Answer from the drawing. Dimensions are ordinates in mm from the lowest x, y and z of the part. A direction names the side the tool comes from. Round coordinates to 2 decimals unless told otherwise and drop trailing zeros. Loops run counter-clockwise (first coordinate to the right, second up) from the corner with the lowest first, then second, coordinate; pieces in that order, holes last.
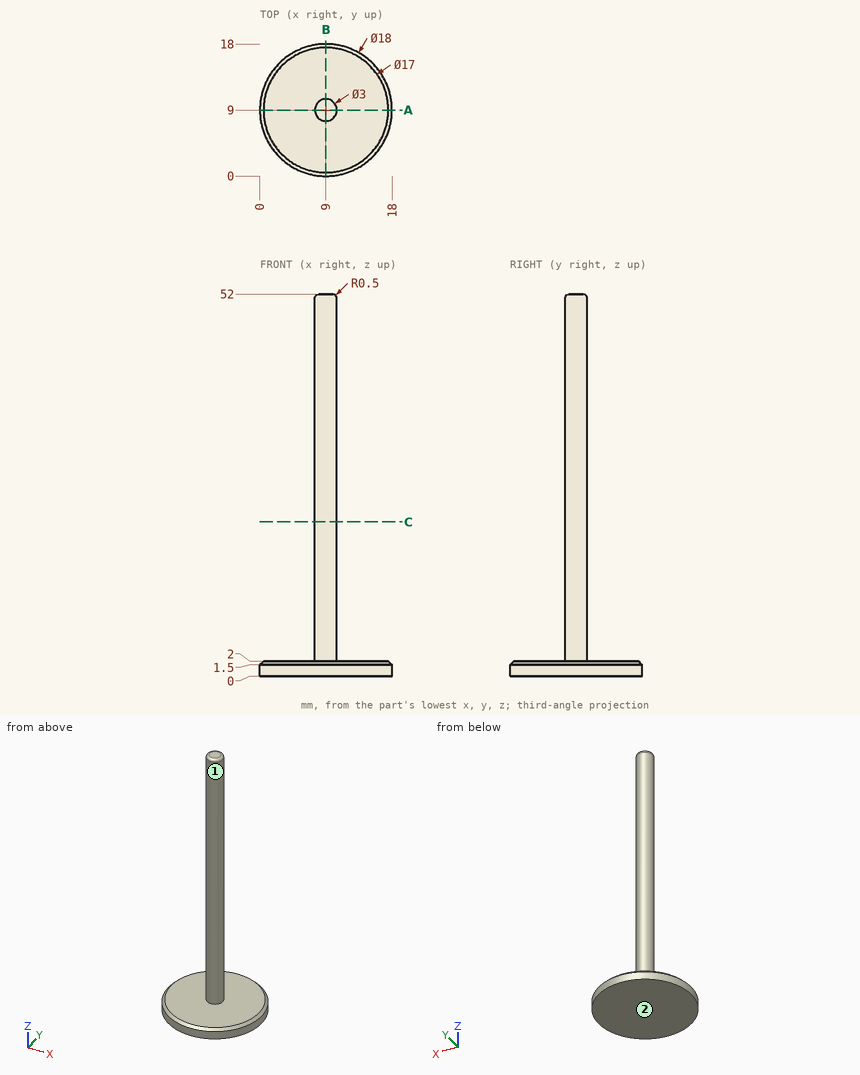
Item 1: Straight lines are drawn through the part: line 1 (Z direction, x = 6, y = 6); line 2 (X direction, y = 8.25, z = 35.5); line 3 (Y direction, x = 8, z = 14). For each, find the intervals that lie inside material, in ascending order.
Item 2: Each of these flat-tipped pins is pushed along its axis until it touches: P1, Ø5, axis at x = 8, z = 26.5, coming from the +Y side; P2, Ø6, axis at y = 10, z = 19, coming from the +X side; P3, Ø6, axis at y = 15, z = 31.5, coming from the +X side; P4, Ø4, axis at x = 10.5, y = 14.5, coming from the -Z side. Where does it stop, or does it pass through?
Item 3: Section C-C, the plane z = 21 is taken. Give the vertices of the cut face in (x, y).
Item 4: Section A-A, the plane y = 9 is taken. Give the vertices of the cut face in (x, z), plus the area to 3 significant figures.
Item 5: For the marked faces 1 and 2, determine the directions among +Z, -Z, +X, -X, +Y, -Y from which every point of the face is accessible in a straight line to the end or side of a thin tool.
Answer below:
1. line 1: z = 0 to 2
1. line 2: x = 7.7 to 10.3
1. line 3: y = 7.88 to 10.12
2. P1: stops at y = 10.5
2. P2: stops at x = 10.5
2. P3: passes through
2. P4: stops at z = 0
3. outline: circle Ø3 at (9, 9)
4. outline: (0, 0) - (18, 0) - (18, 1.5) - (17.5, 2) - (10.5, 2) - (10.5, 51.5) arc R0.5 ccw to (10, 52) - (8, 52) arc R0.5 ccw to (7.5, 51.5) - (7.5, 2) - (0.5, 2) - (0, 1.5) - close
4. area: 186 mm2
5. face 1: +Z
5. face 2: -Z, +X, -X, +Y, -Y
